Input: part model. Units: mm. Frame: model coordinates. Face numbers are marked on the shaded views. A direction names the side the tool comes from. Give positions to 0.01 mm unless a question says otherwise; leave off trailing zeros. Loops run counter-clockwise (first coordinate to the right, second up) from the corner with the lowest first, then second, coordinate; pieces in that order, holes last. Notation, with made-up numbers: (52, 14.25) - (68, 14.25) arc R31 ccw to (68, 52.25) - close; hole circle Ø7 at (64, 74). An arc over 180 degrees is marked (long way). Answer as a JSON object with one key per item and string values.
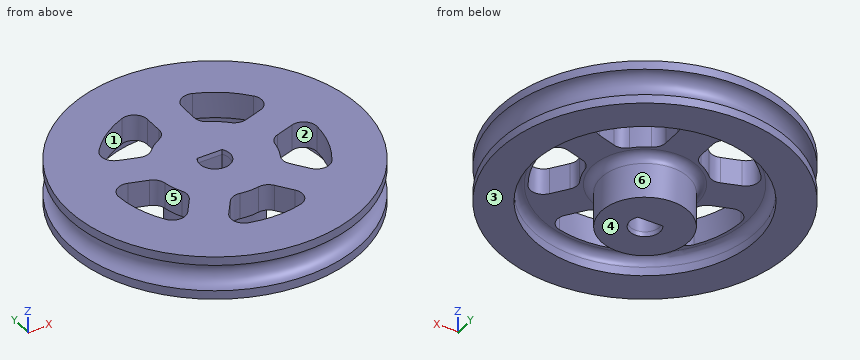
from build123d import *
from OCP.BRepFilletAPI import BRepFilletAPI_MakeChamfer

# Parameters (mm, degrees)
SKETCH7_R           = 12.75
CUT_EXTRUDE3_DEPTH  = 2
SKETCH8_R           = 5
BOSS_EXTRUDE1_DEPTH = 5
CUT_EXTRUDE4_DEPTH  = 26.002499875
FILLET1_R           = 1
CHAMFER1_SIZE       = 0.5
CHAMFER1_SIZE2      = 0.08816349
CHAMFER2_SIZE       = 0.5
CHAMFER2_SIZE2      = 0.08816349
CUT_EXTRUDE7_DEPTH  = 25.210018587
FILLET3_R           = 1.5


with BuildPart() as part:
    # Sketch3 → Revolve1 (revolve)
    with BuildSketch(Plane(origin=(0, 0, 0), x_dir=(1, 0, 0), z_dir=(0, 1, 0)), mode=Mode.PRIVATE) as revolve1_sk:
        with BuildLine():
            Line((0, -2.5), (0, 2.5))
            Line((0, 2.5), (-16.75, 2.5))
            Line((-16.75, 2.5), (-16.75, 1.5))
            ThreePointArc((-16.75, 1.5), (-15.25, 0), (-16.75, -1.5))
            Line((-16.75, -1.5), (-16.75, -2.5))
            Line((-16.75, -2.5), (0, -2.5))
        make_face()
    revolve(revolve1_sk.sketch.rotate(Axis((0, 0, 2.5), (0, 0, -1)), 180), axis=Axis((0, 0, 2.5), (0, 0, -1)))

    # Sketch7 → Cut-Extrude3 (cut)
    with BuildSketch(Plane.XY.offset(-2.5)):
        Circle(SKETCH7_R)
    extrude(amount=CUT_EXTRUDE3_DEPTH, mode=Mode.SUBTRACT)

    # Sketch8 → Boss-Extrude1 (add)
    with BuildSketch(Plane.XY.offset(-0.5)):
        Circle(SKETCH8_R)
    extrude(amount=-BOSS_EXTRUDE1_DEPTH)

    # Sketch6 → Cut-Extrude4 (cut, through all)
    with BuildSketch(Plane.XY.offset(-5.5)):
        with BuildLine():
            Line((-1.382931669, 0.9), (1.382931669, 0.9))
            ThreePointArc((1.382931669, 0.9), (0, -1.65), (-1.382931669, 0.9))
        make_face()
    extrude(amount=CUT_EXTRUDE4_DEPTH, mode=Mode.SUBTRACT)

    # Fillet1
    fillet1_edges = [part.edges().sort_by_distance(p)[0] for p in [
        (-12.75, 0, -0.5),
        (-5, 0, -0.5),
    ]]
    fillet(fillet1_edges, radius=FILLET1_R)

    # Chamfer1: one chamfer whose edges measure the first distance from different faces: ONE call of the kernel's chamfer builder (chamfer() names one face for all edges)
    chamfer1_edges_1 = [part.edges().sort_by_distance(p)[0] for p in [
        (0, -1.65, -5.5),
    ]]
    chamfer1_side_1 = [part.faces().sort_by_distance(p)[0] for p in [
        (0, -1.65, -1.5),
    ]]
    chamfer1_edges_2 = [part.edges().sort_by_distance(p)[0] for p in [
        (0, 0.9, -5.5),
    ]]
    chamfer1_side_2 = [part.faces().sort_by_distance(p)[0] for p in [
        (0, 0.9, -1.5),
    ]]
    chamfer1 = BRepFilletAPI_MakeChamfer(part.part.solid().wrapped)
    for e in chamfer1_edges_1:
        chamfer1.Add(CHAMFER1_SIZE, CHAMFER1_SIZE2, e.wrapped, chamfer1_side_1[0].wrapped)  # the first distance lies on this face
    for e in chamfer1_edges_2:
        chamfer1.Add(CHAMFER1_SIZE, CHAMFER1_SIZE2, e.wrapped, chamfer1_side_2[0].wrapped)  # the first distance lies on this face
    add(Compound.cast(chamfer1.Shape()), mode=Mode.REPLACE)

    # Chamfer2: one chamfer whose edges measure the first distance from different faces: ONE call of the kernel's chamfer builder (chamfer() names one face for all edges)
    chamfer2_edges_1 = [part.edges().sort_by_distance(p)[0] for p in [
        (0, 0.9, 2.5),
    ]]
    chamfer2_side_1 = [part.faces().sort_by_distance(p)[0] for p in [
        (0, 0.9, -1.25),
    ]]
    chamfer2_edges_2 = [part.edges().sort_by_distance(p)[0] for p in [
        (0, -1.65, 2.5),
    ]]
    chamfer2_side_2 = [part.faces().sort_by_distance(p)[0] for p in [
        (0, -1.65, -1.25),
    ]]
    chamfer2 = BRepFilletAPI_MakeChamfer(part.part.solid().wrapped)
    for e in chamfer2_edges_1:
        chamfer2.Add(CHAMFER2_SIZE, CHAMFER2_SIZE2, e.wrapped, chamfer2_side_1[0].wrapped)  # the first distance lies on this face
    for e in chamfer2_edges_2:
        chamfer2.Add(CHAMFER2_SIZE, CHAMFER2_SIZE2, e.wrapped, chamfer2_side_2[0].wrapped)  # the first distance lies on this face
    add(Compound.cast(chamfer2.Shape()), mode=Mode.REPLACE)

    # Sketch11 → Cut-Extrude7 (cut, through all)
    with BuildSketch(Plane(origin=(0, 0, -0.5), x_dir=(-1, 0, 0), z_dir=(0, 0, -1))):
        with BuildLine():
            Line((-2, 6.053150006), (-2, 11.197795542))
            ThreePointArc((-2, 11.197795542), (-6.686057245, 9.202568311), (-10.03170243, 5.362422155))
            Line((-10.03170243, 5.362422155), (-5.138853769, 3.772639254))
            ThreePointArc((-5.138853769, 3.772639254), (-3.747130983, 5.157483339), (-2, 6.053150006))
        make_face()
        with BuildLine():
            ThreePointArc((10.03170243, 5.362422155), (6.686057245, 9.202568311), (2, 11.197795542))
            Line((2, 11.197795542), (2, 6.053150006))
            ThreePointArc((2, 6.053150006), (3.747130983, 5.157483339), (5.138853769, 3.772639254))
            Line((5.138853769, 3.772639254), (10.03170243, 5.362422155))
        make_face()
        with BuildLine():
            Line((-6.374921746, -0.031586811), (-11.267770407, 1.558196089))
            ThreePointArc((-11.267770407, 1.558196089), (-10.818267873, -3.515068311), (-8.199933067, -7.883636388))
            Line((-8.199933067, -7.883636388), (-5.175986292, -3.72153072))
            ThreePointArc((-5.175986292, -3.72153072), (-6.062985291, -1.969983339), (-6.374921746, -0.031586811))
        make_face()
        with BuildLine():
            ThreePointArc((11.375, 0), (11.348160939, 0.780940657), (11.267770407, 1.558196089))
            Line((11.267770407, 1.558196089), (6.374921746, -0.031586811))
            ThreePointArc((6.374921746, -0.031586811), (6.062985291, -1.969983339), (5.175986292, -3.72153072))
            Line((5.175986292, -3.72153072), (8.199933067, -7.883636388))
            ThreePointArc((8.199933067, -7.883636388), (10.551418474, -4.249493286), (11.375, 0))
        make_face()
        with BuildLine():
            Line((-1.939918315, -6.072671729), (-4.963865089, -10.234777398))
            ThreePointArc((-4.963865089, -10.234777398), (0, -11.375), (4.963865089, -10.234777398))
            Line((4.963865089, -10.234777398), (1.939918315, -6.072671729))
            ThreePointArc((1.939918315, -6.072671729), (0, -6.375), (-1.939918315, -6.072671729))
        make_face()
    extrude(amount=-CUT_EXTRUDE7_DEPTH, mode=Mode.SUBTRACT)

    # Fillet3
    fillet3_edges = [part.edges().sort_by_distance(p)[0] for p in [
        (-5.138853769, 3.772639254, 1),
        (-2, 6.053150006, 1),
        (-2, 11.197795542, 1),
        (-10.03170243, 5.362422155, 1),
        (6.374921746, -0.031586811, 1),
        (5.175986292, -3.72153072, 1),
        (8.199933067, -7.883636388, 1),
        (11.267770407, 1.558196089, 1),
        (-5.175986292, -3.72153072, 1),
        (-6.374921746, -0.031586811, 1),
        (-11.267770407, 1.558196089, 1),
        (-8.199933067, -7.883636388, 1),
        (1.939918315, -6.072671729, 1),
        (-1.939918315, -6.072671729, 1),
        (-4.963865089, -10.234777398, 1),
        (4.963865089, -10.234777398, 1),
        (2, 6.053150006, 1),
        (5.138853769, 3.772639254, 1),
        (10.03170243, 5.362422155, 1),
        (2, 11.197795542, 1),
    ]]
    fillet(fillet3_edges, radius=FILLET3_R)


solid = part.part
Item 1: Cut plane B-B (z = -3.75). Return loops of the section in (x, y).
Geometry check:
{"outline": "circle Ø10 at (0, 0); hole (-1.38, 0.9) arc R1.65 ccw (long way) to (1.38, 0.9) - close"}
Item 2: Material intervals for line 1 (Y direction, x = 0, z = -1.75); line 2 (Y direction, x = 1.5, z = -2); line 3 (Y direction, x = 4.5, z = -1.25), sorted ascending. Write a range as [from, to].
Geometry check:
{"line 1": "y = [-16.75, -12.75], [-5, -1.65], [0.9, 5], [12.75, 16.75]", "line 2": "y = [-16.68, -12.66], [-4.77, -0.69], [0.69, 4.77], [12.66, 16.68]", "line 3": "y = [-15.27, -11.9], [-2.25, 2.25], [11.9, 15.27]"}
Item 3: Mould query, pull axis Y, two halves, no side actions, for the marked faces 1, 2 and 3. Classes: released by +Y, released by -Y, zero draft, split by the parting line, or undercut.
Geometry check:
{"face 1": "undercut", "face 2": "undercut", "face 3": "zero draft"}
Item 4: Access query for the marked faces 4, 5 and 6. Directions: +Z, -Z, +X, -X, +Y, -Y. A direction counts if a zero-diameter tool reaches every point of the face in a straight line with its end or side. Return the directions, or none.
Geometry check:
{"face 4": "-Z, +X, -X, +Y, -Y", "face 5": "+Z, -Z", "face 6": "-Z"}
Item 5: Cut plane A-A (x = 0). Give the number of separate pieces and of enclosed holes in the cut face, then the cut area to 3 significant figures.
Geometry check:
{"separate pieces": "3", "enclosed holes": "0", "area": "125 mm2"}
Item 6: Contact query for flat-ended pins moving along their axis: P1, Ø12, axis at x = -11, y = -10, coming from the -Z side; P2, Ø4, axis at x = -2.5, z = -1, coming from the +Y side; P3, Ø1.7, axis at y = 8.5, z = 1, coming from the +X side. Output: stop coordinate, or through.
Geometry check:
{"P1": "stops at z = -2.5", "P2": "stops at y = 16.74", "P3": "stops at x = 14.82"}
